Job drawing, mm, ordinate dimensions from the low corner. One solid piece. A direction names the side the tool comes from. Round coordinates to 2 decimals unless told otherwise and drop trailing zeros. Loops run counter-clockwise (first coordinate to the right, second up) from the corner with the lowest first, then second, coordinate; pieces in that order, holes last. Notation, with made-up numbers: M -19.5,75 L -1.5,75 A23 ccw -1.5,92 Z; hole C 64.25,84 d5. An arc over 180 degrees is marked long. Write each question's results on one line, items separated by ' | '. Start each with the question number.
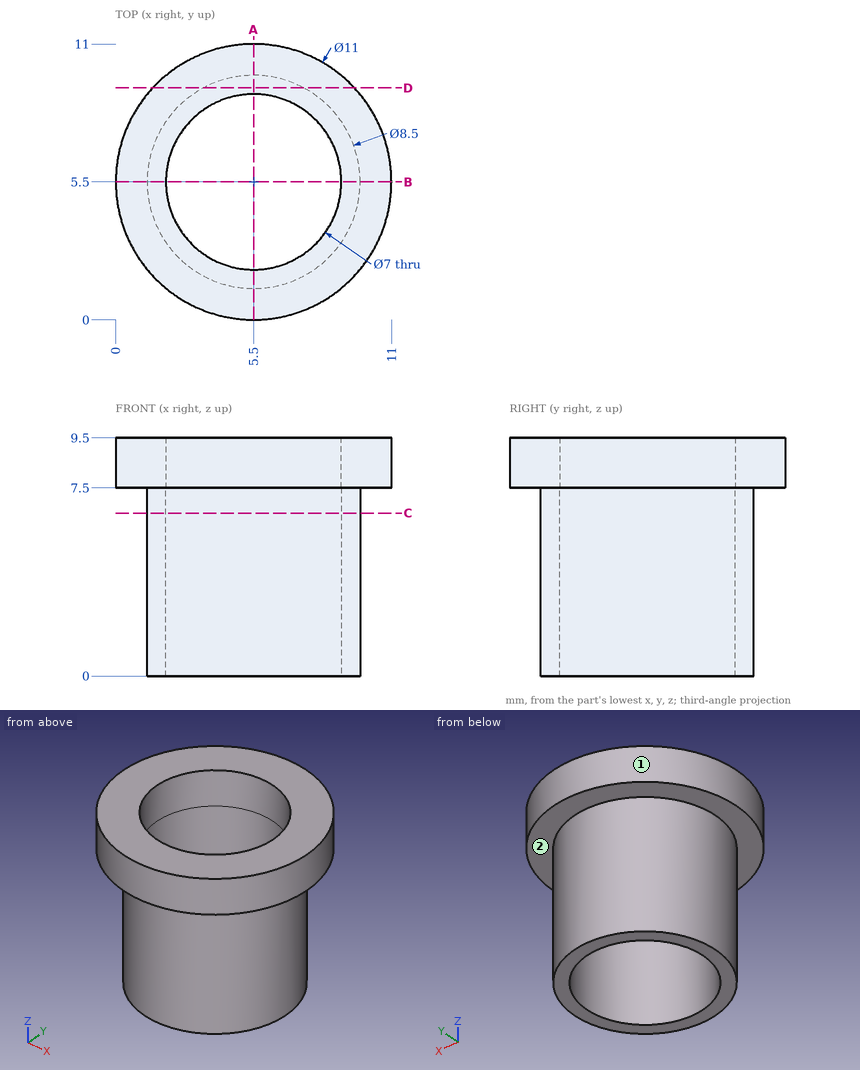
Item 1: Saw through at A-A, the plane x = 5.5. Give the cut face in (y, z), then the cut area to 4 significant figures.
Item 2: Drill centre lines: line 1 along Y through (x, z) = (5.5, 8.9); line 2 along Y through (x, z) = (5.5, 5); line 3 along Z through (x, y) = (3, 10). Where is each one in solid material? Low to high. Write a range as [from, to].
Item 3: Drop flat-ended pins along their axis: pin 1 (3 mm diameter, centred on y = 7.5, z = 7.5, fed in from +X); pin 2 (1.5 mm diameter, centred on y = 1.5, z = 5.5, fed in from -X); pin 3 (4 mm diameter, centred on x = 3, z = 8, fed in from +Y). Give the stop position or say it passes through.
Item 4: Saw through at C-C, the plane z = 6.5. Give the cut face in (x, y), then the cut area to 3 significant figures.
Item 5: Tool access for the marked faces 1 and 2: list every direction of +Z, -Z, +X, -X, +Y, -Y with a clear straight run to the whole face (end or side of a thin tool).
Item 6: Saw through at D-D, the plane y = 9.25. Give the cut face in (x, z).
Working result:
1) outline: M 0,7.5 L 1.25,7.5 L 1.25,0 L 2,0 L 2,9.5 L 0,9.5 Z; M 9,0 L 9.75,0 L 9.75,7.5 L 11,7.5 L 11,9.5 L 9,9.5 Z | area: 19.25 mm²
2) line 1: y = [0, 2], [9, 11] | line 2: y = [1.25, 2], [9, 9.75] | line 3: z = [7.5, 9.5]
3) pin 1: stops at x = 10.98 | pin 2: stops at x = 2.76 | pin 3: stops at y = 10.98
4) outline: C 5.5,5.5 d8.5; hole C 5.5,5.5 d7 | area: 18.3 mm²
5) face 1: +Z, -Z | face 2: -Z
6) outline: M 1.48,7.5 L 3.5,7.5 L 3.5,0 L 7.5,0 L 7.5,7.5 L 9.52,7.5 L 9.52,9.5 L 1.48,9.5 Z
